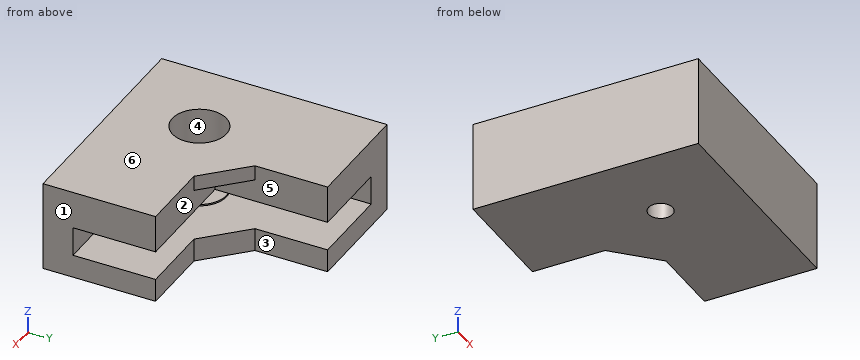
from build123d import *

# Parameters (mm, degrees)
F0_W     = 4
F0_H     = 15
F0_W_2   = 11
F0_H_2   = 11
F0_R     = 3.6
F0_H_3   = 4
F0_R_2   = 1.6
F1_DEPTH = 12
F2_START = 3.1
F2_DEPTH = 3.9
F3_START = 5
F3_DEPTH = 5
F4_START = 3.3
F4_DEPTH = 19.2


# Not quite as in the source:
# - a feature names something its author has since deleted; it is built from what else it names


with BuildPart() as f1:
    # F0 (on Top) → F1 (new body)
    with BuildSketch(Plane.XY):
        with Locations((-13, 7.5)):
            Rectangle(F0_W, F0_H)
        Polygon((-11, 0), (0, 0), (0, 5.31885653), (0, 15), (-7, 15), (-11, 15), align=None)
        Polygon((0, -11), (15, -11), (15, -7), (15, 0), (5.31885653, 0), (0, 0), align=None)
        Polygon((2.9605122421, -15), (15, -15), (15, -11), (0, -11), (0, -15), align=None)
        with Locations((-5.5, -5.5)):
            Rectangle(F0_W_2, F0_H_2)
        with Locations((-4.3933982822, -4.3933982822)):
            Circle(F0_R, mode=Mode.SUBTRACT)
        Polygon((0, 5.31885653), (0, 0), (5.31885653, 0), align=None)
        with Locations((-13, -13)):
            Rectangle(F0_W, F0_H_3)
        Polygon((-15, -11), (-11, -11), (-11, 0), (-15, 0), (-15, -7), align=None)
        with Locations((-5.5, -13)):
            Rectangle(F0_W_2, F0_H_3)
        with Locations((-4.3933982822, -4.3933982822)):
            Circle(F0_R)
        with Locations((-4.3933982822, -4.3933982822)):
            Circle(F0_R_2, mode=Mode.SUBTRACT)
    extrude(amount=F1_DEPTH)

    # F0 (on Top) → F2 (cut)
    with BuildSketch(Plane.XY.offset(F2_START)):
        Polygon((0, -11), (15, -11), (15, -7), (15, 0), (5.31885653, 0), (0, 0), align=None)
        with Locations((-5.5, -5.5)):
            Rectangle(F0_W_2, F0_H_2)
        with Locations((-4.3933982822, -4.3933982822)):
            Circle(F0_R, mode=Mode.SUBTRACT)
        Polygon((-11, 0), (0, 0), (0, 5.31885653), (0, 15), (-7, 15), (-11, 15), align=None)
        Polygon((0, 5.31885653), (0, 0), (5.31885653, 0), align=None)
    extrude(amount=F2_DEPTH, mode=Mode.SUBTRACT)

    # F0 (on Top) → F3 (cut)
    with BuildSketch(Plane.XY.offset(F3_START)):
        Polygon((0, 5.31885653), (0, 0), (5.31885653, 0), align=None)
    extrude(amount=F3_DEPTH, mode=Mode.SUBTRACT)

    # F0 (on Top) → F4 (cut)
    with BuildSketch(Plane.XY.offset(F4_START)):
        with Locations((-4.3933982822, -4.3933982822)):
            Circle(F0_R)
        with Locations((-4.3933982822, -4.3933982822)):
            Circle(F0_R_2, mode=Mode.SUBTRACT)
    extrude(amount=F4_DEPTH, mode=Mode.SUBTRACT)


solid = f1.part
Read the model definition and answer for the solid it produces. Units are mm, in the model's axes. Face numbers are marked on the shaded views. A direction names the side the tool comes from. Coordinates: 2 decimals unless noted, no trailing zeros. Order: outer loops, then holes, each group sorted by start corner. A loop starts at its lowest first (then second) coordinate and runs counter-clockwise, first axis right, second up. Notation, with made-up numbers: (0.5, 56) - (19.5, 56) arc R37 cw to (19.5, 94) - close; hole circle Ø3 at (-4.5, 36). An arc over 180 degrees is marked (long way). Use one line per item in the form item = value.
(1) Section A-A, the plane y = 12.75 is taken. Give the vertices of the cut face in (x, z), then the cut area to 3 significant figures.
Computed values:
outline = (-15, 0) - (0, 0) - (0, 3.1) - (-11, 3.1) - (-11, 7) - (0, 7) - (0, 12) - (-15, 12) - close
area = 137 mm²
(2) Section C-C, the plane y = -6.5 is taken. Give the vertices of the cut face in (x, z), then the cut area to 3 significant figures.
Computed values:
outline = (-15, 0) - (15, 0) - (15, 3.1) - (-1.47, 3.1) - (-1.47, 3.3) - (-7.31, 3.3) - (-7.31, 3.1) - (-11, 3.1) - (-11, 7) - (-7.31, 7) - (-7.31, 12) - (-15, 12) - close; (-1.47, 7) - (15, 7) - (15, 12) - (-1.47, 12) - close
area = 231 mm²
(3) Given pin 1 Ø3.5 at (y, z) = (8, 2.5) entering from +X; pin 2 Ø2.5 at (x, z) = (11, 1.5) entering from +Y, each flat-ended and moving along its own axis, determine where each tip first touches the part or whether it passes through.
Computed values:
pin_1 = 0
pin_2 = 0
(4) Which of the six approach directions +Z, -Z, +X, -X, +Y, -Y give full straight-line access (tool end or side, diameter ignored) to the marked faces 1, 2 and 3?
Computed values:
face_1 = +Z, -Z, +X, +Y, -Y
face_2 = +X, +Y
face_3 = +Z, -Z, +X, +Y
(5) For a pull along X with two mould halves and no side action, classify the marked faces 4, 5 and 6 as pulls with the +X half, pulls with the -X half, needs draft (parallel to the pull), parting line crosses it, or undercut.
Computed values:
face_4 = undercut
face_5 = pulls with the +X half
face_6 = needs draft
(6) Straight lines are drawn through the part: L1, parallel to Z at x = -0.5, y = -4.75; L2, parallel to Z at x = -6.75, y = -2.75; L3, parallel to Y at x = 6, z = 5.5. For each, find the intervals that lie inside material, in ascending order.
Computed values:
L1 = 0 to 3.1, 7 to 12
L2 = 0 to 3.3
L3 = -15 to -11
(7) Section B-B, the plane x = -5.5 is taken. Give the vertices of the cut face in (y, z), then the cut area to 3 significant figures.
Computed values:
outline = (-15, 0) - (-5.55, 0) - (-5.55, 3.3) - (-7.82, 3.3) - (-7.82, 3.1) - (-11, 3.1) - (-11, 7) - (-7.82, 7) - (-7.82, 12) - (-15, 12) - close; (-3.24, 0) - (15, 0) - (15, 3.1) - (-0.97, 3.1) - (-0.97, 3.3) - (-3.24, 3.3) - close; (-0.97, 7) - (15, 7) - (15, 12) - (-0.97, 12) - close
area = 218 mm²
(8) Section D-D, the plane x = -9 is taken. Give the vertices of the cut face in (y, z).
Computed values:
outline = (-15, 0) - (15, 0) - (15, 3.1) - (-11, 3.1) - (-11, 7) - (15, 7) - (15, 12) - (-15, 12) - close
